Autodesk Inventor part; units mm, degrees
ref_plane "YZ Plane" through (0, 0, 0) normal (1, 0, 0) x (0, 1, 0)
ref_plane "XZ Plane" through (0, 0, 0) normal (0, 1, 0) x (-1, 0, 0)
ref_plane "XY Plane" through (0, 0, 0) normal (0, 0, 1) x (1, 0, 0)
sketch "Sketch1" plane through (0, 0, 0) normal (0, 0, 1) x (1, 0, 0)
  line L0 (0, 0) -> (41, 0)
  line L1 (41, 0) -> (41, 41)
  line L2 (41, 41) -> (0, 41)
  line L3 (0, 41) -> (0, 0)
  line L4 (20.5, 20.5) -> (20.5, 36)
  line L5 (20.5, 36) -> (5, 36)
  circle A0 centre (5, 36) radius 1.725
  circle A1 centre (36, 36) radius 1.725
  circle A2 centre (5, 5) radius 1.725
  circle A3 centre (36, 5) radius 1.725
  circle A4 centre (20.5, 20.5) radius 17.5
  line L6 (0, 36) -> (-3.81, 36)
  circle A5 centre (-3.81, 36) radius 2.2225
  line L7 (41, 36) -> (44.81, 36)
  circle A6 centre (44.81, 36) radius 2.2225
  line L8 (0, 41) -> (-3.81, 41)
  line L9 (0, 36) -> (0, 30.9962)
  line L10 (0, 30.9962) -> (-3.81, 30.9962)
  arc A7 (-3.81, 41) -> (-3.81, 30.9962) centre (-3.81, 35.9981) ccw
  line L11 (41, 41) -> (44.81, 41)
  line L12 (41, 36) -> (41, 30.9962)
  line L13 (41, 30.9962) -> (44.81, 30.9962)
  arc A8 (44.81, 30.9962) -> (44.81, 41) centre (44.81, 35.9981) ccw
  dimension "d0" = 41
  dimension "d1" = 41
  dimension "d2" = 15.5
  dimension "d3" = 15.5
  dimension "d4" = 3.45
  dimension "d7" = 31
  dimension "d10" = 31
  dimension "d13" = 35
  dimension "d14" = 3.81
  dimension "d15" = 4.445
  dimension "d16" = 3.81
  dimension "d17" = 4.445
  dimension "d18" = 5.0038
  dimension "d19" = 5.0038
extrude "Extrusion1" add sketch "Sketch1" along normal blind 2.54
fillet "Fillet1" radius 7.9375 2 edges at (0, 30.9962, 1.27) (41, 30.9962, 1.27)
properties part number "FanMount"
For this review, take the finished solid that the model builds, in its own axes (mm). A direction names the side the tool comes from. Coordinates: 2 decimals unless noted, no trailing zeros. Write each loop counter-clockwise with the first axis right and the second up, starting at its lowest first coordinate (ties: lowest second). Pieces come first, ordered by that corner, then holes.
(1) For pin 1 Ø2.5 at (x, y) = (-3.81, 36) entering from -Z; pin 2 Ø1 at (y, z) = (32.5, 0.5) entering from -X, all flat-tipped, find the tip position at first contact; note any pin that passes through.
(2) Add section D-D on z = 0.55. Count the separate pieces of the cut face and the enclosed holes in it, then the cut area to 3 significant figures.
(3) Add section A-A on x = 20.5. Give the boundary of the cut face in (y, z), then the cut area to 3 significant figures.
(4) Add section B-B on y = 36. Give the boundary of the cut face in (x, z) (1 decimal).
(5) Tool access review of faces 1 (the face through (5.8, 37.53, 1.25)), 2 (the face through (41, 12, 1)), 3 (the face through (0, 12, 1)): name each direction out of +Z, -Z, +X, -X, +Y, -Y from which nothing blocks a thin tool from reaching the whole face with its end or side.
(6) The part is to be moulded in two halves that separate along X. For faces 4 (the face through (-8.76, 36.71, 1.25)), 5 (the face through (42.59, 35.9, 1.25)), 6 (the face through (20, 39, 0)), 7 (the face through (7.602, 8.673, 1.252)), say which applies: +X half, -X half, draft (parallel to the pull), parting line (faces both ways), or undercut.
(7) Add section C-C on x = 5. Give the boundary of the cut face in (y, z) (3 decimals).
(8) Wall thickness on probe 1 along Y at (x, z) = (20.5, 2.2); probe 2 along Y at (x, z) = (36, 1.3) (3 decimals): over which ranges is each line inside the solid? List them lowest first.
Answer sheet:
1. pin 1: passes through
1. pin 2: stops at x = -7.81
2. separate pieces: 1
2. enclosed holes: 7
2. area: 825 mm2
3. outline: (0, 0) - (3, 0) - (3, 2.54) - (0, 2.54) - close; (38, 0) - (41, 0) - (41, 2.54) - (38, 2.54) - close
3. area: 15.2 mm2
4. outline: (-8.8, 0) - (-6, 0) - (-6, 2.5) - (-8.8, 2.5) - close; (-1.6, 0) - (3.3, 0) - (3.3, 2.5) - (-1.6, 2.5) - close; (6.7, 0) - (12.4, 0) - (12.4, 2.5) - (6.7, 2.5) - close; (28.6, 0) - (34.3, 0) - (34.3, 2.5) - (28.6, 2.5) - close; (37.7, 0) - (42.6, 0) - (42.6, 2.5) - (37.7, 2.5) - close; (47, 0) - (49.8, 0) - (49.8, 2.5) - (47, 2.5) - close
5. face 1: +Z, -Z
5. face 2: +Z, -Z, +X, -Y
5. face 3: +Z, -Z, -X, -Y
6. face 4: -X half
6. face 5: undercut
6. face 6: draft
6. face 7: undercut
7. outline: (0, 0) - (3.275, 0) - (3.275, 2.54) - (0, 2.54) - close; (6.725, 0) - (12.376, 0) - (12.376, 2.54) - (6.725, 2.54) - close; (28.624, 0) - (34.275, 0) - (34.275, 2.54) - (28.624, 2.54) - close; (37.725, 0) - (41, 0) - (41, 2.54) - (37.725, 2.54) - close
8. probe 1: y = 0 to 3, 38 to 41
8. probe 2: y = 0 to 3.275, 6.725 to 12.376, 28.624 to 34.275, 37.725 to 41
